Input: part model. Units: mm. Frame: model coordinates. Face numbers are marked on the shaded views. A direction names the side the tool comes from. Round coordinates to 2 decimals unless told otherwise and drop trailing zeros. Order: outer loops, then holes, each group sorted by start corner. A loop starts at its lowest first (then second) coordinate and runs counter-clockwise, first axis right, second up.
Item 1: Cut plane A-A on x = 58. Output: boundary loops of the cut face in (y, z).
Item 2: Cut plane C-C on z = 613. Output: boundary loops of the cut face in (x, y), then the cut area to 3 significant figures.
Item 3: First-contact query: pin 1 (7.5 mm diameter, centred on x = 29, z = 109, fed in from -Y); pin 2 (8 mm diameter, centred on y = -52.5, z = 740.5, fed in from -X); pin 3 (12 mm diameter, centred on y = -25.5, z = 670, fed in from +X); pin 4 (12 mm diameter, centred on x = 57, z = 105.5, fed in from -Y). Flat tips, straight axial feed; report the tip coordinate or a pass-through.
Item 4: Reachability of the marked faces 1, 2 and 3 from +Z, -Z, +X, -X, +Y, -Y: full face, straight path, thin tool, end or side. Return the list, or none.
Item 5: Cut plane B-B on y = -77. Output: boundary loops of the cut face in (x, z), then the cut area to 3 significant figures.
Item 6: Cut plane D-D on x = 110.5. Output: boundary loops of the cut face in (y, z), then the cut area to 3 significant figures.
Item 7: Line query: L1, parallel to X at y = -3, z = 132; L2, parallel to Y at x = 35, z = 827. Output: solid intervals per line, ascending.
```python
from build123d import *

# Parameters (mm, degrees)
F0_W     = 101.6
F0_H     = 101.6
F1_DEPTH = 1016
F4_W     = 152.4
F4_H     = 152.4
F5_DEPTH = 127
F6_W     = 203.2
F6_H     = 203.2
F7_DEPTH = 101.6


with BuildPart() as f1:
    # F0 (on Top) → F1 (new body)
    with BuildSketch(Plane.XY):
        with Locations((50.8, -50.8)):
            Rectangle(F0_W, F0_H)
    extrude(amount=F1_DEPTH)

    # F4 (on Top) → F5 (join)
    with BuildSketch(Plane.XY):
        with Locations((50.8, -50.8)):
            Rectangle(F4_W, F4_H)
    extrude(amount=F5_DEPTH)

    # F6 (on Top) → F7 (join)
    with BuildSketch(Plane.XY):
        with Locations((50.8, -50.8)):
            Rectangle(F6_W, F6_H)
    extrude(amount=F7_DEPTH)


solid = f1.part
```
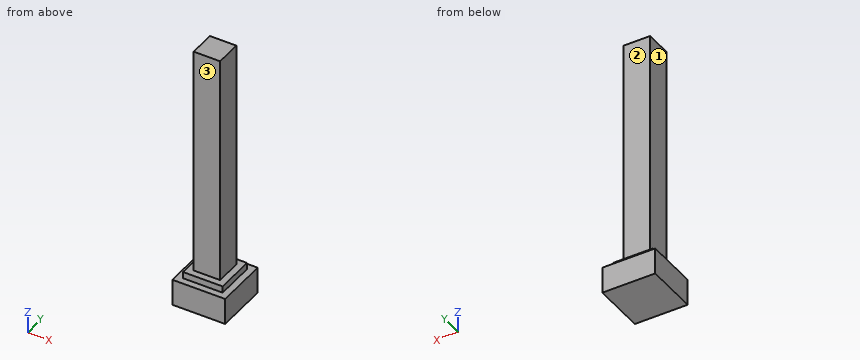
From the geometry:
1. outline: (-152.4, 0) - (50.8, 0) - (50.8, 101.6) - (25.4, 101.6) - (25.4, 127) - (0, 127) - (0, 1016) - (-101.6, 1016) - (-101.6, 127) - (-127, 127) - (-127, 101.6) - (-152.4, 101.6) - close
2. outline: (0, -101.6) - (101.6, -101.6) - (101.6, 0) - (0, 0) - close
2. area: 10,300 mm2
3. pin 1: stops at y = -127
3. pin 2: stops at x = 0
3. pin 3: stops at x = 101.6
3. pin 4: stops at y = -152.4
4. face 1: +Z, -X, +Y, -Y
4. face 2: +Z, +X, -X, +Y
4. face 3: +Z, +X, -X, -Y
5. outline: (-50.8, 0) - (152.4, 0) - (152.4, 101.6) - (127, 101.6) - (127, 127) - (101.6, 127) - (101.6, 1016) - (0, 1016) - (0, 127) - (-25.4, 127) - (-25.4, 101.6) - (-50.8, 101.6) - close
5. area: 115,000 mm2
6. outline: (-152.4, 0) - (50.8, 0) - (50.8, 101.6) - (25.4, 101.6) - (25.4, 127) - (-127, 127) - (-127, 101.6) - (-152.4, 101.6) - close
6. area: 24,500 mm2
7. L1: x = 0 to 101.6
7. L2: y = -101.6 to 0
